Source: CAD feature listing. Evaluate the final solid. Frame: model axes, mm. Give positions to 0.01 mm unless a question says otherwise; leave off trailing zeros. Loops run counter-clockwise (first coordinate to the right, second up) from the corner with the lowest first, then second, coordinate; pieces in that order, holes last. Notation, with made-up numbers: (17, -17.75) - (36, -17.75) arc R30 cw to (36, 20.25) - close; hole circle Ø8 at (-31, -14.75). An arc over 180 degrees is marked (long way). Put each result on its own line as item: value.
```python
from build123d import *

# Parameters (mm, degrees)
SKETCH1_W           = 92.6
SKETCH1_H           = 300
BOSS_EXTRUDE1_DEPTH = 2
SKETCH2_R           = 2.25
SKETCH2_W           = 8.48
SKETCH2_H           = 53
SKETCH2_H_2         = 50
CUT_EXTRUDE5_DEPTH  = 10
FILLET3_R           = 2
SKETCH4_R           = 1.85
CUT_EXTRUDE6_DEPTH  = 10
SKETCH5_R           = 1.85
CUT_EXTRUDE7_DEPTH  = 5
SKETCH6_W           = 48
SKETCH6_H           = 60
CUT_EXTRUDE8_DEPTH  = 10


with BuildPart() as part:
    # Sketch1 → Boss-Extrude1 (new body)
    with BuildSketch(Plane.XY):
        Rectangle(SKETCH1_W, SKETCH1_H)
    extrude(amount=BOSS_EXTRUDE1_DEPTH)

    # Sketch2 → Cut-Extrude5 (cut)
    with BuildSketch(Plane.XY):
        with Locations((-42.06, 75)):
            Circle(SKETCH2_R)
        with Locations((42.06, 125)):
            Circle(SKETCH2_R)
        with Locations((42.06, 25)):
            Circle(SKETCH2_R)
        with Locations((42.06, -75)):
            Circle(SKETCH2_R)
        with Locations((-42.06, -25)):
            Circle(SKETCH2_R)
        with Locations((-42.06, -125)):
            Circle(SKETCH2_R)
        with Locations((-42.06, 123.5)):
            Rectangle(SKETCH2_W, SKETCH2_H)
        with Locations((42.06, 75)):
            Rectangle(SKETCH2_W, SKETCH2_H_2)
        with Locations((42.06, -25)):
            Rectangle(SKETCH2_W, SKETCH2_H_2)
        with Locations((-42.06, 25)):
            Rectangle(SKETCH2_W, SKETCH2_H)
        with Locations((-42.06, -75)):
            Rectangle(SKETCH2_W, SKETCH2_H)
        with Locations((42.06, -125)):
            Rectangle(SKETCH2_W, SKETCH2_H_2)
    extrude(amount=CUT_EXTRUDE5_DEPTH, mode=Mode.SUBTRACT)

    # Fillet3
    fillet3_edges = [part.edges().sort_by_distance(p)[0] for p in [
        (46.3, -100, 1),
        (37.82, -100, 1),
        (37.82, -150, 1),
        (46.3, 50, 1),
        (46.3, 100, 1),
        (37.82, 100, 1),
        (37.82, 50, 1),
        (-46.3, -48.5, 1),
        (-46.3, -101.5, 1),
        (-37.82, -101.5, 1),
        (-37.82, -48.5, 1),
        (37.82, 0, 1),
        (37.82, -50, 1),
        (46.3, -50, 1),
        (46.3, 0, 1),
        (46.3, 150, 1),
        (-46.3, -150, 1),
        (-46.3, 51.5, 1),
        (-46.3, -1.5, 1),
        (-37.82, -1.5, 1),
        (-37.82, 51.5, 1),
        (-46.3, 97, 1),
        (-37.82, 97, 1),
        (-37.82, 150, 1),
    ]]
    fillet(fillet3_edges, radius=FILLET3_R)

    # Sketch4 → Cut-Extrude6 (cut)
    with BuildSketch(Plane(origin=(0, 0, 0), x_dir=(-1, 0, 0), z_dir=(0, 0, -1))):
        with Locations((-25, -142)):
            Circle(SKETCH4_R)
        with Locations((25, -142)):
            Circle(SKETCH4_R)
        with Locations((32, 142)):
            Circle(SKETCH4_R)
        with Locations((-32, 142)):
            Circle(SKETCH4_R)
    extrude(amount=-CUT_EXTRUDE6_DEPTH, mode=Mode.SUBTRACT)

    # Sketch5 → Cut-Extrude7 (cut)
    with BuildSketch(Plane(origin=(0, 0, 0), x_dir=(-1, 0, 0), z_dir=(0, 0, -1))):
        with Locations((-27, -103)):
            Circle(SKETCH5_R)
        with Locations((27, -103)):
            Circle(SKETCH5_R)
        with Locations((-27, -7)):
            Circle(SKETCH5_R)
        with Locations((27, -7)):
            Circle(SKETCH5_R)
        with Locations((-32, 37)):
            Circle(SKETCH5_R)
        with Locations((32, 37)):
            Circle(SKETCH5_R)
        with Locations((-28.75, 58)):
            Circle(SKETCH5_R)
        with Locations((28.75, 80.08)):
            Circle(SKETCH5_R)
        with Locations((-28.75, 100)):
            Circle(SKETCH5_R)
    extrude(amount=-CUT_EXTRUDE7_DEPTH, mode=Mode.SUBTRACT)

    # Sketch6 → Cut-Extrude8 (cut)
    with BuildSketch(Plane(origin=(0, 0, 0), x_dir=(-1, 0, 0), z_dir=(0, 0, -1))):
        with Locations((1.1, 78.923300873)):
            Rectangle(SKETCH6_W, SKETCH6_H)
    extrude(amount=-CUT_EXTRUDE8_DEPTH, mode=Mode.SUBTRACT)


solid = part.part
```
1) Section query A-A, the plane y = 105. Output: boundary loops of the cut face in (x, z), plus the area to 3 significant figures.
Check result:
outline: (-37.82, 0) - (-25.1, 0) - (-25.1, 2) - (-37.82, 2) - close; (22.9, 0) - (46.3, 0) - (46.3, 2) - (22.9, 2) - close
area: 72.2 mm²
2) Section query B-B, the plane z = 1.15. State how many separate pieces and enclosed holes the cut face has, plus the area to 3 significant figures.
Check result:
separate pieces: 1
enclosed holes: 20
area: 22,000 mm²
3) Pin query (flat end, axial travel): P1, Ø1, axis at y = -117.5, z = 1.5, coming from the +X side; P2, Ø1, axis at x = -42.5, z = 1.5, coming from the +Y side. Return the tip coordinate at first contact, or that it passes through.
Check result:
P1: x = 37.82
P2: y = 97
4) Material intervals for line 1 along Y through (x, z) = (42.06, 1.45); line 2 along X through (y, z) = (125, 0.75); line 3 along X through (y, z) = (81, 1), sorted ascending. Write a range as [from, to].
Check result:
line 1: [-100, -77.25], [-72.75, -50], [0, 22.75], [27.25, 50], [100, 122.75], [127.25, 150]
line 2: [-37.82, 39.81], [44.31, 46.3]
line 3: [-46.3, -30.36], [-27.14, -25.1], [22.9, 37.82]
